Could you check a few things on this model? Use its own coordinates, in mm. A direction names the side the tool comes from. Coordinates: 2 decimals unless noted, no trailing zeros. Loops run counter-clockwise (first coordinate to the right, second up) from the corner with the lowest first, then second, coordinate; pieces in that order, holes last. Notation, with made-up numbers: M 5,24 L 45,24 A25 cw 45,38 Z; hole C 46,-27 d9. An arc over 180 degrees is marked long. Write each question's results on one line, items separated by ' | '.
```python
from build123d import *

# Parameters (mm, degrees)
BOSS_EXTRUDE1_DEPTH   = 4
F_6_32_TAPPED_HOLE1_D = 2.7051
SKETCH4_R             = 3.044
CUT_EXTRUDE1_DEPTH    = 1.905
SKETCH5_R             = 1.75
CUT_EXTRUDE2_DEPTH    = 3.095


with BuildPart() as part:
    # Sketch1 → Boss-Extrude1 (new body)
    with BuildSketch(Plane(origin=(0, 0, 0), x_dir=(1, 0, 0), z_dir=(0, 1, 0))):
        with BuildLine():
            ThreePointArc((2.505986433, 2.505986433), (5.111833916, -3.531413722), (2.866848356, -9.712083716))
            ThreePointArc((2.866848356, -9.712083716), (1.571428319, -10.663233366), (0, -11))
            ThreePointArc((0, -11), (-7.778174593, -7.778174593), (-11, 0))
            ThreePointArc((-11, 0), (-10.663233366, 1.571428319), (-9.712083716, 2.866848356))
            ThreePointArc((-9.712083716, 2.866848356), (-3.531413722, 5.111833916), (2.505986433, 2.505986433))
        make_face()
    extrude(amount=BOSS_EXTRUDE1_DEPTH)

    # #6-32 Tapped Hole1 (through all)
    with Locations(Plane(origin=(0, 0, 0), x_dir=(-1, 0, 0), z_dir=(0, -1, 0))):
        with Locations((8, 0), (0, -8)):
            Hole(F_6_32_TAPPED_HOLE1_D / 2)

    # Sketch4 → Cut-Extrude1 (cut)
    with BuildSketch(Plane.XZ):
        Circle(SKETCH4_R)
    extrude(amount=-CUT_EXTRUDE1_DEPTH, mode=Mode.SUBTRACT)

    # Sketch5 → Cut-Extrude2 (cut, through all)
    with BuildSketch(Plane.XZ.offset(-1.905)):
        Circle(SKETCH5_R)
    extrude(amount=-CUT_EXTRUDE2_DEPTH, mode=Mode.SUBTRACT)


solid = part.part
```
(1) Imagine slicing it at A-A, the plane y = 2.2. List the corners of the cut face in (x, z) for me.
Reported:
outline: M -11,0 A3.83 ccw -9.71,-2.87 A8.91 ccw 2.87,9.71 A3.83 ccw 0,11 A11 ccw Z; hole C -8,0 d2.71; hole C 0,0 d3.5; hole C 0,8 d2.71
(2) Will these pins go through, and if not, where does the flat tip stop? P1, Ø1, axis at x = -9.5, y = 3, coming from the +Z side; P2, Ø2, axis at y = 0.5, z = -2, coming from the +X side; P3, Ø2, axis at y = 1, z = 4, coming from the -X side.
Reported:
P1: stops at z = 6.32 | P2: stops at x = 3.72 | P3: stops at x = -10.58
(3) If we mould it in two halves opening along X, with no side actions, what happens to faces 3 (the cylindrical face through (1.617, 2.938, -0.67)), 4 (the flat face through (-3, 4, 3)), 5 (the cylindrical face through (-7.692, 1.972, 7.863))? For each: released by +X, released by -X, zero draft, split by the parting line, or undercut.
Reported:
face 3: undercut | face 4: zero draft | face 5: released by -X
(4) Which directions (+Z, -Z, +X, -X, +Y, -Y) give clear straight access to the entire face, cutting with the end or side of a thin tool? Please do faces 1 (the cylindrical face through (2.903, 0.939, 0.914)), 2 (the cylindrical face through (1.592, 1.972, 10.654)).
Reported:
face 1: -Y | face 2: +Z, +X, +Y, -Y
(5) Imagine slicing it at B-B, the plane x = 1. List the corners of the cut face in (y, z) for me (3 decimals), and give its area (3 significant figures).
Reported:
outline: M 0,-3.716 L 4,-3.716 L 4,-1.436 L 1.905,-1.436 L 1.905,-2.875 L 0,-2.875 Z; M 0,2.875 L 1.905,2.875 L 1.905,1.436 L 4,1.436 L 4,7.089 L 0,7.089 Z; M 0,8.911 L 4,8.911 L 4,10.867 L 0,10.867 Z | area: 34.1 mm2
(6) Imagine slicing it at C-C, the plane y = 0.6. List the corners of the cut face in (x, z) for me.
Reported:
outline: M -11,0 A3.83 ccw -9.71,-2.87 A8.91 ccw 2.87,9.71 A3.83 ccw 0,11 A11 ccw Z; hole C -8,0 d2.71; hole C 0,0 d6.09; hole C 0,8 d2.71
(7) Please list where these lines run through material, in increasing order: probe 1 along Z at (x, y) = (0.25, 3.55); probe 2 along Z at (x, y) = (0, 0.75); probe 3 along Z at (x, y) = (-8, 2.55). Write a range as from..to.
Reported:
probe 1: z = -4.14..-1.73, 1.73..6.67, 9.33..10.99 | probe 2: z = -4.27..-3.04, 3.04..6.65, 9.35..11 | probe 3: z = -4.06..-1.35, 1.35..7.55
(8) Imagine slicing it at D-D, the plane z = -0.75. List the corners of the cut face in (x, y) for me (3 decimals).
Reported:
outline: M -10.926,0 L -9.126,0 L -9.126,4 L -10.926,4 Z; M -6.874,0 L -2.95,0 L -2.95,1.905 L -1.581,1.905 L -1.581,4 L -6.874,4 Z; M 1.581,1.905 L 2.95,1.905 L 2.95,0 L 3.87,0 L 3.87,4 L 1.581,4 Z
